Verification items for the finished model (mm, model axes). A direction names the side the tool comes from. Coordinates: 2 decimals unless noted, no trailing zeros. Loops run counter-clockwise (first coordinate to the right, second up) from the corner with the lowest first, then second, coordinate; pieces in that order, holes last. Notation, with made-up numbers: (76, -26) - (121, -26) arc R14 cw to (121, -18) - close; hole circle Ø1 at (87, -17.75). An arc over 180 degrees is marked (long way). One line per item, written item: value. Start each with the question number.
(1) Section check C-C (z = 449.5). Record the boundary of the cut face in (x, y).
(2) Draft check along X on faces 1 (the face through (-20, 0, 338)), 2 (the face through (18, 0, 319)), 3 (the face through (-18, 0, 337)), 4 (the face through (0, -20, 336)). Enter one of: +X half, -X half, draft (parallel to the pull), parting line (faces both ways), or undercut.
(3) Section check B-B (y = 10). Record the boundary of the cut face in (x, z), plus the area to 3 significant figures.
(4) Section check A-A (x = 6.5). Record the boundary of the cut face in (y, z).
(5) Set-up check for faces 5 (the face through (0, -18, 336)), 6 (the face through (20, 0, 318)): record each of +Z, -Z, +X, -X, +Y, -Y from which the full face is reachable in a straight line by a thin tool's end or side.
(6) Thickness scan on probe 1 along Y at (x, z) = (-16.5, 431.5); probe 2 along Y at (x, z) = (-15, 484). Record the ranges inside material, lowest first. Write a range as [from, to].
Autodesk Inventor part; units mm, degrees
ref_plane "Piano iniziale" through (0, 0, 0) normal (0, 0, 1) x (1, 0, 0)
ref_plane "Piano finale" through (0, 0, 685.5) normal (0, 0, 1) x (1, 0, 0)
ref_plane "YZ Plane" through (0, 0, 0) normal (1, 0, 0) x (0, 1, 0)
ref_plane "Piano iniziale" through (0, 0, 0) normal (0, 0, 1) x (1, 0, 0)
ref_plane "Piano finale" through (0, 0, 685.5) normal (0, 0, 1) x (1, 0, 0)
sketch "Schizzo" plane through (0, 0, 0) normal (0, 0, 1) x (1, 0, 0)
  line L0 (-20, -16) -> (-20, 16)
  line L1 (-16, 20) -> (16, 20)
  line L2 (20, 16) -> (20, -16)
  line L3 (16, -20) -> (-16, -20)
  arc A0 (-20, -16) -> (-16, -20) centre (-16, -16) ccw
  arc A1 (20, 16) -> (16, 20) centre (16, 16) ccw
  arc A2 (-16, 20) -> (-20, 16) centre (-16, 16) ccw
  arc A3 (16, -20) -> (20, -16) centre (16, -16) ccw
  arc A4 (-16, 18) -> (-18, 16) centre (-16, 16) ccw
  line L4 (-16, 18) -> (16, 18)
  arc A5 (18, 16) -> (16, 18) centre (16, 16) ccw
  line L5 (18, 16) -> (18, -16)
  arc A6 (16, -18) -> (18, -16) centre (16, -16) ccw
  line L6 (16, -18) -> (-16, -18)
  arc A7 (-18, -16) -> (-16, -18) centre (-16, -16) ccw
  line L7 (-18, -16) -> (-18, 16)
  line L8 (0, 29.1598) -> (0, -29.1598) construction
  line L9 (-29.1598, 0) -> (29.1598, 0) construction
  dimension "d7" = 4
  dimension "d9" = 40
  dimension "d11" = 40
  dimension "d12" = 2
  dimension "d15" = 20
  dimension "d16" = 20
extrude "Corpo" add sketch "Schizzo" along normal up to surface (685.5 mm away) from surface at 0
sketch "Sketch3" plane through (0, 0, 0) normal (0, 0, 1) x (1, 0, 0)
  line L0 (0, 0) -> (10, 0)
ref_plane "Work Plane3" through (0, 0, 0) normal (0, -1, 0) x (1, 0, 0)
sketch "Sketch4" plane through (0, 0, 0) normal (0, -1, 0) x (1, 0, 0)
  line L0 (-2, 0) -> (12, 0)
  line L1 (-2, 685.5) -> (12, 685.5)
  dimension "d18" = 685.5
sketch "Schizzo5" plane through (-16, -20, 0) normal (0, -1, 0) x (1, 0, 0)
  line L0 (-4, 0) -> (-4, 685.5)
  line L1 (-4, 685.5) -> (0, 685.5)
  line L2 (-4, 685.5) -> (40.4052, 641.0948)
  line L3 (-4, 685.5) -> (58.7984, 685.5) construction
  line L4 (40.4052, 641.0948) -> (40.4052, 697.863)
  line L5 (36, 0) -> (36, 685.5)
  line L6 (40.4052, 697.863) -> (-4, 685.5)
  point P0 (16, 0)
  dimension "d19" = 45
extrude "Estrusione2" cut sketch "Schizzo5" against normal up to next
equation "\"d7\" = G_IR"
equation "\"d9\" = G_W"
equation "\"d11\" = G_H"
equation "\"d12\" = G_T"
equation "\"d15\" = 0.5 * d9"
equation "\"d16\" = 0.5 * d11"
equation "\"d3\" = G_L"
equation "\"G_W\" = 40"
equation "\"G_H\" = 40"
equation "\"G_T\" = 2"
equation "\"G_IR\" = 4"
equation "\"G_L\" = d18"
equation "\"G_OFFSET_START\" = 0"
equation "\"G_OFFSET_END\" = 0"
equation "\"d14\" = G_OFFSET_END + B_L"
equation "\"B_L\" = 685.5"
properties part number "ISO 10799-2 - 40x40x2 - 685,5" material "Acciaio, Dolce"
Responses:
1. outline: (-20, -16) arc R4 ccw to (-16, -20) - (16, -20) arc R4 ccw to (20, -16) - (20, 16) arc R4 ccw to (16, 20) - (-16, 20) arc R4 ccw to (-20, 16) - close; hole (-18, -16) arc R2 ccw to (-16, -18) - (16, -18) arc R2 ccw to (18, -16) - (18, 16) arc R2 ccw to (16, 18) - (-16, 18) arc R2 ccw to (-18, 16) - close
2. face 1: -X half
2. face 2: undercut
2. face 3: undercut
2. face 4: draft
3. outline: (-20, 0) - (-18, 0) - (-18, 683.5) - (-20, 685.5) - close; (18, 0) - (20, 0) - (20, 645.5) - (18, 647.5) - close
3. area: 2,660 mm²
4. outline: (-20, 0) - (-18, 0) - (-18, 659) - (-20, 659) - close; (18, 0) - (20, 0) - (20, 659) - (18, 659) - close
5. face 5: +Z, -Z
5. face 6: +Z, -Z, +X, +Y, -Y
6. probe 1: y = [-19.97, -17.94], [17.94, 19.97]
6. probe 2: y = [-20, -18], [18, 20]
